from build123d import *

# Parameters (mm, degrees)
F0_R     = 0.85
F1_DEPTH = 5


with BuildPart() as f1:
    # F0 (on Front) → F1 (new body)
    with BuildSketch(Plane.XZ):
        with BuildLine():
            Line((-2.25, 0), (0, 0))
            Line((0, 0), (2.25, 0))
            ThreePointArc((2.25, 0), (2.957107, 0.292893), (3.25, 1))
            Line((3.25, 1), (3.25, 2.25))
            ThreePointArc((3.25, 2.25), (2.957107, 2.957107), (2.25, 3.25))
            Line((2.25, 3.25), (0, 3.25))
            Line((0, 3.25), (-2.25, 3.25))
            ThreePointArc((-2.25, 3.25), (-2.957107, 2.957107), (-3.25, 2.25))
            Line((-3.25, 2.25), (-3.25, 1))
            ThreePointArc((-3.25, 1), (-2.957107, 0.292893), (-2.25, 0))
        make_face()
        with Locations((-1.75, 1.625)):
            Circle(F0_R, mode=Mode.SUBTRACT)
        with Locations((1.75, 1.625)):
            Circle(F0_R, mode=Mode.SUBTRACT)
    extrude(amount=F1_DEPTH)


solid = f1.part
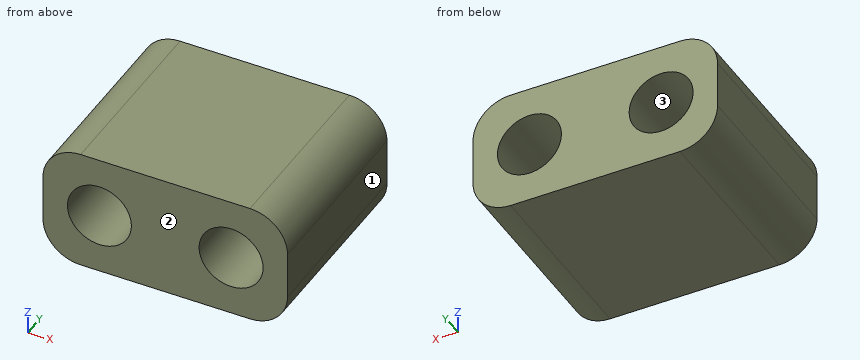
Build history of the part. All positions in model axes, mm. Face numbers are marked on the shaded views. Give positions to 0.01 mm unless a question says otherwise; leave off trailing zeros. Loops run counter-clockwise (first coordinate to the right, second up) from the corner with the lowest first, then second, coordinate; pieces in that order, holes last. Notation, with made-up numbers: (89, -6.75) -> (130, -6.75) arc R31 cw to (130, 24.25) -> close; hole circle Ø1 at (9.25, 55.25). An arc over 180 degrees is marked (long way). Answer in a Markdown table with one row per item.
Item 1: Mould opens along X. For the marked faces 1, 2 and 3 say: pulls with the +X half, pulls with the -X half, needs draft (parallel to the pull), parting line crosses it, or undercut.
Findings below:
| item | result |
|---|---|
| face 1 | pulls with the +X half |
| face 2 | needs draft |
| face 3 | undercut |
Item 2: Slice it at A-A on x = -1.75. Write the cut outline in (y, z) (3 decimals).
Findings below:
| item | result |
|---|---|
| outline | (-5, 0) -> (0, 0) -> (0, 0.775) -> (-5, 0.775) -> close; (-5, 2.475) -> (0, 2.475) -> (0, 3.25) -> (-5, 3.25) -> close |
Item 3: Slice it at C-C on x = 2.75. Write the cut outline in (y, z).
Findings below:
| item | result |
|---|---|
| outline | (-5, 0.13) -> (0, 0.13) -> (0, 3.12) -> (-5, 3.12) -> close |
Item 4: Slice it at B-B on y = -0.9. Write the cut outline in (x, z) (3 decimals).
Findings below:
| item | result |
|---|---|
| outline | (-3.25, 1) arc R1 ccw to (-2.25, 0) -> (2.25, 0) arc R1 ccw to (3.25, 1) -> (3.25, 2.25) arc R1 ccw to (2.25, 3.25) -> (-2.25, 3.25) arc R1 ccw to (-3.25, 2.25) -> close; hole circle Ø1.7 at (-1.75, 1.625); hole circle Ø1.7 at (1.75, 1.625) |
Item 5: Probe line 1 along Z through (x, y) = (1.75, -2.3) (3 decimals); line 2 along X through (y, z) = (-2.2, 1.4); line 3 along X through (y, z) = (-3.4, 2). List the from-to ranges inside material, lowest first. Write a range as [from, to].
Findings below:
| item | result |
|---|---|
| line 1 | z = [0, 0.775], [2.475, 3.25] |
| line 2 | x = [-3.25, -2.57], [-0.93, 0.93], [2.57, 3.25] |
| line 3 | x = [-3.25, -2.51], [-0.99, 0.99], [2.51, 3.25] |
